Autodesk Inventor part; units mm, degrees
ref_plane "YZ Plane" through (0, 0, 0) normal (1, 0, 0) x (0, 1, 0)
ref_plane "XZ Plane" through (0, 0, 0) normal (0, 1, 0) x (-1, 0, 0)
ref_plane "XY Plane" through (0, 0, 0) normal (0, 0, 1) x (1, 0, 0)
sketch "Sketch1" plane through (0, 0, 0) normal (0, 1, 0) x (-1, 0, 0)
  line L0 (-21, -21) -> (21, -21)
  line L1 (21, -21) -> (21, 21)
  line L2 (21, 21) -> (-21, 21)
  line L3 (-21, 21) -> (-21, -21)
  line L4 (-21, -21) -> (21, 21) construction
  line L5 (21, -21) -> (-21, 21) construction
  circle A0 centre (0, 0) radius 75
  circle A1 centre (50, 0) radius 12.5
  circle A2 centre (50, 0) radius 14.5
  line L6 (50, 0) -> (0, 0) construction
  dimension "d0" = 42
  dimension "d1" = 42
  dimension "d2" = 150
  dimension "d3" = 50
  dimension "d4" = 2
  dimension "d5" = 25
extrude "Extrusion1" add sketch "Sketch1" along normal blind 10 contours A0 | A1 | A2
extrude "Extrusion2" add sketch "Sketch1" along normal blind 50 from surface at 10 contours A2
sketch "Sketch2" plane through (0, 10, 0) normal (0, 1, 0) x (1, 0, 0)
  circle A0 centre (-50, 0) radius 14.5
  line L0 (21, 21) -> (21, -21)
  line L1 (21, -21) -> (-21, -21)
  line L2 (-21, -21) -> (-21, 21)
  line L3 (-21, 21) -> (21, 21)
  circle A1 centre (0, 0) radius 75
  circle A2 centre (0, 0) radius 70
  dimension "d10" = 5
extrude "Extrusion3" add sketch "Sketch2" along normal blind 50 contours A1
pattern_circular "Circular Pattern1" count 8 over 360 about axis through (0, 0, 0) along (0, 1, 0) of "Extrusion2"
properties part number "bottom"
Can you work these out from the model? Positions are in its coordinate system, mm. A direction names the side the tool comes from. Give positions to 0.01 mm unless a question says otherwise; leave off trailing zeros. Order: outer loops, then holes, each group sorted by start corner. A loop starts at its lowest first (then second) coordinate and runs counter-clockwise, first axis right, second up. Notation, with made-up numbers: M 33.25,51 L 85.25,51 A15 ccw 85.25,66 Z; hole C 89.25,5.5 d11. An arc over 180 degrees is marked long. One line per question, with ' | ' between items.
Item 1: Suppose I cut it at B-B, the plane z = 55. Write out the boundary of the cut face in (x, y).
Answer block:
outline: M -50.99,0 L 50.99,0 L 50.99,60 L 43.3,60 L 43.3,10 L 13.61,10 L 13.61,60 L 11.46,60 L 11.46,10 L -11.46,10 L -11.46,60 L -13.61,60 L -13.61,10 L -43.3,10 L -43.3,60 L -50.99,60 Z
Item 2: Suppose I cut it at A-A, the plane y = 26.5. Give the number of separate pieces and of enclosed holes in the cut face, then the cut area to 3 significant figures.
Answer block:
separate pieces: 9 | enclosed holes: 9 | area: 3,630 mm2
Item 3: Suppose I cut it at D-D, the plane y = 8. Write out the boundary of the cut face in (x, z).
Answer block:
outline: C 0,0 d150; hole M -21,-21 L 21,-21 L 21,21 L -21,21 Z
Item 4: We'd pull the mould along Z, two halves only. Please class faces 1 (the face through (-35, 10, 36)), 2 (the face through (-30, 60, 47)): released by +Z, released by -Z, zero draft, split by the parting line, or undercut.
Answer block:
face 1: undercut | face 2: zero draft
Item 5: Suppose I cut it at C-C, the plane x = -56.5. Write out the boundary of the cut face in (y, z).
Answer block:
outline: M 0,-49.32 L 60,-49.32 L 60,-41.32 L 10,-41.32 L 10,-12.96 L 60,-12.96 L 60,-10.68 L 10,-10.68 L 10,10.68 L 60,10.68 L 60,12.96 L 10,12.96 L 10,41.32 L 60,41.32 L 60,49.32 L 0,49.32 Z
Item 6: I'm going to push flat-ended pins straight in: pin 1 Ø20 at (x, z) = (-39, 37.5) entering from +Y; pin 2 Ø1.5 at (y, z) = (38.5, 8.5) entering from +X; pin 3 Ø3 at (x, y) = (-7.5, 5) entering from +Z; pin 4 Ø1.5 at (x, y) = (-28, 48.5) entering from +Z. Where does each tip first touch, or does it pass through?
Answer block:
pin 1: stops at y = 60 | pin 2: stops at x = 74.6 | pin 3: stops at z = 74.76 | pin 4: stops at z = 69.87
Item 7: For faces 3 (the face through (47, 60, 30)), 4 (the face through (-21, 5, 0)), 5 (the face through (-35, 10, -35)), which set-ups out of +Z, -Z, +X, -X, +Y, -Y let a thin tool reach every point of the face, with its end or its side?
Answer block:
face 3: +Z, -Z, +X, -X, +Y | face 4: +Y, -Y | face 5: +Y
Item 8: Please list where these lines run through material, in increasing order: L1, parallel to X at y = 14, z = -0.5; L2, parallel to Z at x = 5.5, y = 47; L3, parallel to X at y = 28, z = 59.
Answer block:
L1: x = -75 to -70, -64.49 to -62.49, -37.51 to -35.51, 35.51 to 37.51, 62.49 to 64.49, 70 to 75 | L2: z = -74.8 to -69.78, -63.42 to -61.22, -38.78 to -36.58, 36.58 to 38.78, 61.22 to 63.42, 69.78 to 74.8 | L3: x = -46.3 to -37.67, -11.37 to -8.67, 8.67 to 11.37, 37.67 to 46.3
